Check sheet for the modelled part. Datum: model origin and axes. Units: mm. Coordinates: 2 decimals unless noted, no trailing zeros. Loops run counter-clockwise (first coordinate to the right, second up) from the corner with the lowest first, then second, coordinate; pieces in that order, holes last.
from build123d import *

# Parameters (mm, degrees)
BOSS_EXTRUDE1_DEPTH = 10
SKETCH2_W           = 41.5
SKETCH2_H           = 20.5
CUT_EXTRUDE1_DEPTH  = 20
SKETCH3_R           = 6
CUT_EXTRUDE2_DEPTH  = 510.509568114
SKETCH4_R           = 6
CUT_EXTRUDE3_DEPTH  = 510.509568114
CUT_EXTRUDE4_DEPTH  = 10
SKETCH11_W          = 20.354372897
SKETCH11_H          = 12
SKETCH11_W_2        = 24.350914836
SKETCH11_W_3        = 29.997295682
CUT_EXTRUDE5_DEPTH  = 10
M3_TAPPED_HOLE1_D   = 2.5
M6_TAPPED_HOLE1_D   = 5


with BuildPart() as part:
    # Sketch1 → Boss-Extrude1 (new, symmetric)
    with BuildSketch(Plane.XY):
        with BuildLine():
            Line((50, 360), (310, 360))
            ThreePointArc((310, 360), (345.355339059, 345.355339059), (360, 310))
            Line((360, 310), (360, 50))
            ThreePointArc((360, 50), (345.355339059, 14.644660941), (310, 0))
            Line((310, 0), (50, 0))
            ThreePointArc((50, 0), (14.644660941, 14.644660941), (0, 50))
            Line((0, 50), (0, 310))
            ThreePointArc((0, 310), (14.644660941, 345.355339059), (50, 360))
        make_face()
    extrude(amount=BOSS_EXTRUDE1_DEPTH, both=True)

    # Sketch2 → Cut-Extrude1 (cut)
    with BuildSketch(Plane.XY.offset(10)):
        with Locations((54.25, 295.25)):
            Rectangle(SKETCH2_W, SKETCH2_H)
        with Locations((305.75, 295.25)):
            Rectangle(SKETCH2_W, SKETCH2_H)
        with Locations((305.75, 64.75)):
            Rectangle(SKETCH2_W, SKETCH2_H)
        with Locations((54.25, 64.75)):
            Rectangle(SKETCH2_W, SKETCH2_H)
    extrude(amount=-CUT_EXTRUDE1_DEPTH, mode=Mode.SUBTRACT)

    # Sketch3 → Cut-Extrude2 (cut, through all)
    with BuildSketch(Plane.XY.offset(10)):
        with Locations((92, 295)):
            Circle(SKETCH3_R)
        with Locations((268, 295)):
            Circle(SKETCH3_R)
        with Locations((268, 65)):
            Circle(SKETCH3_R)
        with Locations((92, 65)):
            Circle(SKETCH3_R)
    extrude(amount=-CUT_EXTRUDE2_DEPTH, mode=Mode.SUBTRACT)

    # Sketch4 → Cut-Extrude3 (cut, through all)
    with BuildSketch(Plane.XY.offset(10)):
        with Locations((140, 235)):
            Circle(SKETCH4_R)
        with Locations((220, 235)):
            Circle(SKETCH4_R)
        with Locations((220, 125)):
            Circle(SKETCH4_R)
        with Locations((140, 125)):
            Circle(SKETCH4_R)
    extrude(amount=-CUT_EXTRUDE3_DEPTH, mode=Mode.SUBTRACT)

    # Sketch10 → Cut-Extrude4 (cut)
    with BuildSketch(Plane(origin=(0, 0, -10), x_dir=(-1, 0, 0), z_dir=(0, 0, -1))):
        Polygon((-87.314787143, 291.251829715), (-135.314787143, 231.251829715), (-144.685212857, 238.748170285), (-96.685212857, 298.748170285), align=None)
        Polygon((-263.314787143, 61.251829715), (-215.314787143, 121.251829715), (-224.685212857, 128.748170285), (-272.685212857, 68.748170285), align=None)
        Polygon((-87.314787143, 68.748170285), (-135.314787143, 128.748170285), (-144.685212857, 121.251829715), (-96.685212857, 61.251829715), align=None)
        Polygon((-272.685212857, 291.251829715), (-224.685212857, 231.251829715), (-215.314787143, 238.748170285), (-263.314787143, 298.748170285), align=None)
    extrude(amount=-CUT_EXTRUDE4_DEPTH, mode=Mode.SUBTRACT)

    # Sketch11 → Cut-Extrude5 (cut)
    with BuildSketch(Plane.XY.offset(10)):
        with Locations((81.822813552, 65)):
            Rectangle(SKETCH11_W, SKETCH11_H)
        with Locations((280.175457418, 65)):
            Rectangle(SKETCH11_W_2, SKETCH11_H)
        with Locations((280.175457418, 295)):
            Rectangle(SKETCH11_W_2, SKETCH11_H)
        with Locations((77.001352159, 295)):
            Rectangle(SKETCH11_W_3, SKETCH11_H)
    extrude(amount=-CUT_EXTRUDE5_DEPTH, mode=Mode.SUBTRACT)

    # M3 Tapped Hole1 (through all)
    with Locations(Plane(origin=(135, 150, 10), x_dir=(1, 0, 0), z_dir=(0, 0, 1))):
        with Locations((0, 0), (90, 60), (0, 60), (90, 0)):
            Hole(M3_TAPPED_HOLE1_D / 2)

    # M6 Tapped Hole1 (through all)
    with Locations(Plane(origin=(152.5, 280, 10), x_dir=(1, 0, 0), z_dir=(0, 0, 1))):
        with Locations((0, 0), (55, 0)):
            Hole(M6_TAPPED_HOLE1_D / 2)


solid = part.part
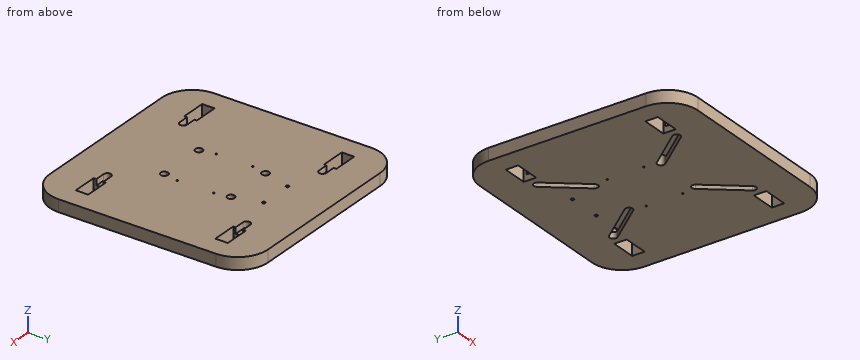
(1) Gauge pin test, flat end, axial feed: P1, Ø6, axis at x = 81.5, y = 296.5, coming from the +Z side. Record the tip position at first contact, or that the pin passes through.
(2) Scan lines: line 1 along X through (y, z) = (150, -1.25); line 2 along X through (y, z) = (295, 4.5); line 3 along Y through (x, z) = (62, -3.5). Record each from-to range of solid material in increasing order.
(3) Section check A-A, the plane x = 44.5. Enter the section's corners in (y, z).
(4) Section check B-B, the plane z = 6.5. Count the separate pieces of the cut face and the enclosed holes in it, plus the area to 3 significant figures.
(5) Section check D-D, the plane y = 28.5. Enter the section's corners in (x, z).
(6) Section check C-C, the plane x = 124.5. Enter the section's corners in (y, z).
Determined:
1. P1: stops at z = 0
2. line 1: x = 0 to 133.75, 136.25 to 223.75, 226.25 to 360
2. line 2: x = 0 to 33.5, 98 to 262, 326.5 to 360
2. line 3: y = 0 to 54.5, 75 to 285, 305.5 to 360
3. outline: (0.3, -10) - (54.5, -10) - (54.5, 10) - (0.3, 10) - close; (75, -10) - (285, -10) - (285, 10) - (75, 10) - close; (305.5, -10) - (359.7, -10) - (359.7, 10) - (305.5, 10) - close
4. separate pieces: 1
4. enclosed holes: 14
4. area: 122,000 mm2
5. outline: (4.86, -10) - (355.14, -10) - (355.14, 10) - (4.86, 10) - close
6. outline: (0, -10) - (96.02, -10) - (96.02, 0) - (115.23, 0) - (115.23, -10) - (244.77, -10) - (244.77, 0) - (263.98, 0) - (263.98, -10) - (360, -10) - (360, 10) - (0, 10) - close
